from build123d import *

# Parameters (mm, degrees)
ESBO_O1_W                  = 30
ESBO_O1_H                  = 10
RESSALTO_EXTRUS_O1_DEPTH   = 13
ESBO_O2_W                  = 30
ESBO_O2_H                  = 3.8
CORTE_EXTRUS_O1_DEPTH      = 10
FILETE1_R                  = 3
CORTE_EXTRUS_O2_DEPTH      = 23.226110771
CORTE_EXTRUS_O2_DEPTH_BACK = 23.226110771
ESBO_O3_W                  = 2.5
ESBO_O3_H                  = 4
ESBO_O4_W                  = 25
ESBO_O4_H                  = 25
RESSALTO_EXTRUS_O2_DEPTH   = 1.5
CHANFRO1_SIZE              = 5
CHANFRO1_SIZE_2            = 8.660254038
CHANFRO2_SIZE              = 7
CHANFRO2_SIZE2             = 4.041451884
ESBO_O5_R                  = 8.5
ESBO_O5_R_2                = 1
CORTE_EXTRUS_O3_DEPTH      = 3
FILETE2_R                  = 4


with BuildPart() as part:
    # Esboço1 → Ressalto-extrusão1 (new body)
    with BuildSketch(Plane.XY):
        Rectangle(ESBO_O1_W, ESBO_O1_H)
    extrude(amount=RESSALTO_EXTRUS_O1_DEPTH)

    # Esboço2 → Corte-extrusão1 (cut)
    with BuildSketch(Plane.XY.offset(13)):
        Rectangle(ESBO_O2_W, ESBO_O2_H)
    extrude(amount=-CORTE_EXTRUS_O1_DEPTH, mode=Mode.SUBTRACT)

    # Filete1
    filete1_edges = [part.edges().sort_by_distance(p)[0] for p in [
        (-15, 3.45, 13),
        (15, 3.45, 13),
        (-15, -3.45, 13),
        (15, -3.45, 13),
    ]]
    fillet(filete1_edges, radius=FILETE1_R)

    # Esboço3 → Corte-extrusão2 (cut, two sides: drawn at the far end of the back side and taken through both)
    with BuildSketch(Plane(origin=(0, 5, 0), x_dir=(1, 0, 0), z_dir=(0, 1, 0)).offset(-CORTE_EXTRUS_O2_DEPTH_BACK)):
        with Locations((9.906768391, -9)):
            Rectangle(ESBO_O3_W, ESBO_O3_H)
        with Locations((-9.906768391, -9)):
            Rectangle(ESBO_O3_W, ESBO_O3_H)
    extrude(amount=CORTE_EXTRUS_O2_DEPTH + CORTE_EXTRUS_O2_DEPTH_BACK, mode=Mode.SUBTRACT)

    # Esboço4 → Ressalto-extrusão2 (add, symmetric)
    with BuildSketch(Plane(origin=(13, 0, 0), x_dir=(0, 0, -1), z_dir=(1, 0, 0))):
        with Locations((12.5, 8.5)):
            Rectangle(ESBO_O4_W, ESBO_O4_H)
    extrude(amount=RESSALTO_EXTRUS_O2_DEPTH, both=True)

    # Chanfro1
    # the kernel refuses this chamfer: 8.660254038, 5 mm, written as the material it adds along each edge
    with BuildSketch(Plane(origin=(11.5, -4, 0), x_dir=(0, -0.9983227437537924, 0.05789386240267202), z_dir=(1, 0, 0))) as chanfro1_piece_1_section:
        Polygon((CHANFRO1_SIZE * 0.998322743754, CHANFRO1_SIZE * 0.0578938624027), (-CHANFRO1_SIZE_2 * 0.0578938624016, CHANFRO1_SIZE_2 * 0.998322743736), (0, 0), align=None)
    chanfro1_piece_1 = extrude(amount=3, mode=Mode.PRIVATE)
    chanfro1_piece_1 = split(chanfro1_piece_1, bisect_by=Plane(origin=(13, -5, -4.055902091), z_dir=(0, 1, 0)), keep=Keep.TOP, mode=Mode.PRIVATE)
    add(chanfro1_piece_1)

    # Chanfro2
    chanfro2_edges = [part.edges().sort_by_distance(p)[0] for p in [
        (13, 5, 0),
    ]]
    chanfro2_side = [part.faces().sort_by_distance(p)[0] for p in [
        (0, 5, 6.301932384),
    ]]
    chamfer(chanfro2_edges, length=CHANFRO2_SIZE, length2=CHANFRO2_SIZE2, reference=chanfro2_side[0])

    # Esboço5 → Corte-extrusão3 (cut)
    with BuildSketch(Plane.ZY.offset(-11.5)):
        with Locations((-12.5, 10)):
            Circle(ESBO_O5_R)
        with Locations((-20.2, 17.7)):
            Circle(ESBO_O5_R_2)
        with Locations((-4.8, 17.7)):
            Circle(ESBO_O5_R_2)
        with Locations((-4.8, 2.3)):
            Circle(ESBO_O5_R_2)
        with Locations((-20.2, 2.3)):
            Circle(ESBO_O5_R_2)
    extrude(amount=-CORTE_EXTRUS_O3_DEPTH, mode=Mode.SUBTRACT)

    # Filete2
    filete2_edges = [part.edges().sort_by_distance(p)[0] for p in [
        (13, 21, 0),
        (13, 21, -25),
        (13, -4, -25),
    ]]
    fillet(filete2_edges, radius=FILETE2_R)


solid = part.part
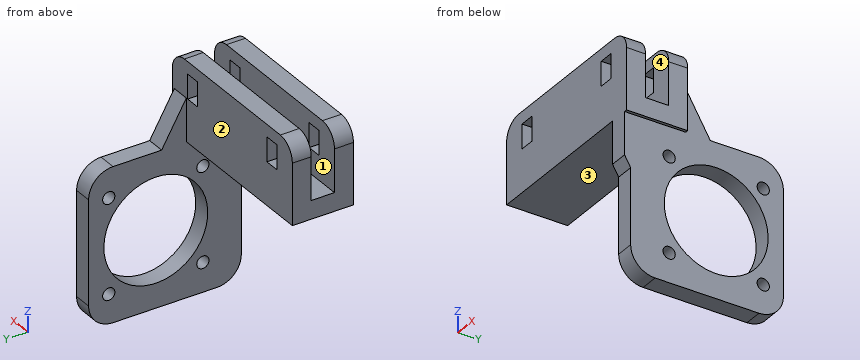
Can you work these out from the model? Positions are in its coordinate system, mm. Face numbers are marked on the shaded views. Round coordinates to 2 decimals unless told otherwise and drop trailing zeros. Loops run counter-clockwise (first coordinate to the right, second up) from the corner with the lowest first, then second, coordinate; pieces in that order, holes last. Notation, with made-up numbers: (40, 89.25) - (68, 89.25) arc R32 cw to (68, 117.25) - close; hole circle Ø11 at (10.25, 25.5). An arc over 180 degrees is marked (long way). Answer in a Markdown table with one row per item. Add a question column.
Q1. We'd pull the mould along Y, two halves only. Please class the marked faces 1, 2, 3 and 4: pulls with the +Y half, pulls with the -Y half, needs draft (parallel to the pull), parting line crosses it, or undercut.
Q2. I need wall thicknesses on L1, parallel to Y at x = -1.5, z = 10.5; L2, parallel to Y at x = 12.7, z = -4.8; L3, parallel to Y at x = 12.75, z = -12.5. Which ranges of each line are inside material? Lowest first, please.
Q3. I want a section at A-A on z = -20.2. List the corners of the cut face in (x, y) for me.
Q4. I want a section at B-B on y = 4.25. List the corners of the cut face in (x, z) for me, and give its area (3 significant figures).
Q5. I want a section at D-D on y = 10. List the corners of the cut face in (x, z) for me.
Q6. I want a section at C-C on z = 7.5. List the corners of the cut face in (x, y) for me, and give its area (3 significant figures).
Q7. For pin 1 Ø3 at (y, z) = (18, -6.5) entering from +X; pin 2 Ø1.5 at (x, y) = (12.5, 12.5) entering from +Z; pin 3 Ø1.6 at (y, z) = (17.7, -4.8) entering from -X; pin 4 Ø1.5 at (x, y) = (0, 1) entering from +Z, each with a flat end and sliding along its axis, tell me the tip position at first contact or that it passes through.
A:
| question | item | result |
|---|---|---|
| 1 | face 1 | undercut |
| 1 | face 2 | pulls with the +Y half |
| 1 | face 3 | needs draft |
| 1 | face 4 | undercut |
| 2 | L1 | -5 to -1.9, 1.9 to 5 |
| 2 | L2 | -5 to 1.3, 3.3 to 6.4, 13.6 to 16.7, 18.7 to 21 |
| 2 | L3 | -4 to 1.5, 18.5 to 21 |
| 3 | outline | (11.5, -4) - (14.5, -4) - (14.5, 1.3) - (11.5, 1.3) - close; (11.5, 3.3) - (14.5, 3.3) - (14.5, 6.4) - (11.5, 6.4) - close; (11.5, 13.6) - (14.5, 13.6) - (14.5, 16.7) - (11.5, 16.7) - close; (11.5, 18.7) - (14.5, 18.7) - (14.5, 21) - (11.5, 21) - close |
| 4 | outline | (-15, 0) - (11.5, 0) - (11.5, -6.24) - (14.5, -6.24) - (14.5, 0) - (15, 0) - (15, 10) arc R3 ccw to (12, 13) - (-12, 13) arc R3 ccw to (-15, 10) - close; (11.5, -25) - (14.5, -25) - (14.5, -18.76) - (11.5, -18.76) - close; hole (-11.16, 7) - (-8.66, 7) - (-8.66, 11) - (-11.16, 11) - close; hole (8.66, 7) - (11.16, 7) - (11.16, 11) - (8.66, 11) - close |
| 4 | area | 404 mm^2 |
| 5 | outline | (11.5, -25) - (14.5, -25) - (14.5, -21) - (11.5, -21) - close; (11.5, -4) - (14.5, -4) - (14.5, 0) - (11.5, 0) - close |
| 6 | outline | (-15, -5) - (-11.16, -5) - (-11.16, -1.9) - (-15, -1.9) - close; (-15, 1.9) - (-11.16, 1.9) - (-11.16, 5) - (-15, 5) - close; (-8.66, -5) - (8.66, -5) - (8.66, -1.9) - (-8.66, -1.9) - close; (-8.66, 1.9) - (8.66, 1.9) - (8.66, 5) - (-8.66, 5) - close; (11.16, -5) - (15, -5) - (15, -1.9) - (11.16, -1.9) - close; (11.16, 1.9) - (15, 1.9) - (15, 5) - (11.16, 5) - close |
| 6 | area | 155 mm^2 |
| 7 | pin 1 | x = 14.5 |
| 7 | pin 2 | z = 0 |
| 7 | pin 3 | through |
| 7 | pin 4 | z = 3 |
